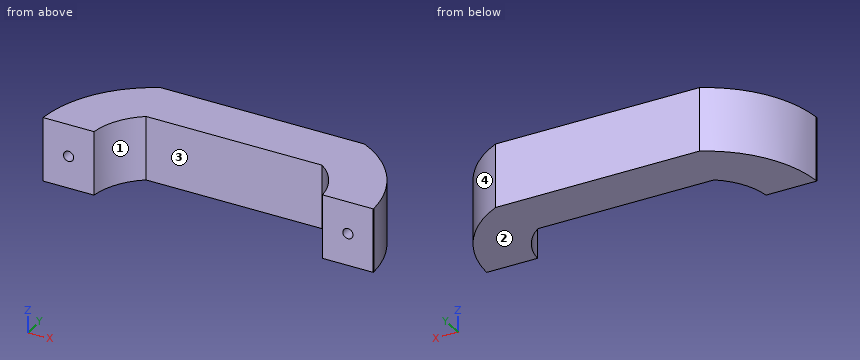
from build123d import *

# Parameters (mm, degrees)
BOSS_EXTRUDE1_DEPTH = 25
SKETCH3_R           = 2
CUT_EXTRUDE1_DEPTH  = 10


with BuildPart() as part:
    # Sketch2 → Boss-Extrude1 (new body)
    with BuildSketch(Plane.XY):
        with BuildLine():
            Line((-34.654096647, 18), (33.564112537, 18))
            Line((33.564112537, 18), (34.654096647, 18))
            ThreePointArc((34.654096647, 18), (41.754772696, 10.113790987), (44.967734696, 0))
            Line((44.967734696, 0), (64.929939713, 0))
            ThreePointArc((64.929939713, 0), (64.983093484, 0.336809111), (64.97700751, 0.677732359))
            ThreePointArc((64.97700751, 0.677732359), (57.505542276, 22.646902561), (40.105840234, 38))
            Line((40.105840234, 38), (33.564112537, 38))
            Line((33.564112537, 38), (-40.105840234, 38))
            ThreePointArc((-40.105840234, 38), (-57.505542276, 22.646902561), (-64.97700751, 0.677732359))
            ThreePointArc((-64.97700751, 0.677732359), (-65.02406211, 0.339344907), (-65.063625193, 0))
            Line((-65.063625193, 0), (-44.967734696, 0))
            ThreePointArc((-44.967734696, 0), (-41.754772696, 10.113790987), (-34.654096647, 18))
        make_face()
    extrude(amount=BOSS_EXTRUDE1_DEPTH)

    # Sketch3 → Cut-Extrude1 (cut)
    with BuildSketch(Plane.XZ):
        with Locations(Location((-55, 12.5, 0), (0, 0, 270))):
            Circle(SKETCH3_R)
        with Locations(Location((55, 12.5, 0), (0, 0, 90))):
            Circle(SKETCH3_R)
    extrude(amount=-CUT_EXTRUDE1_DEPTH, mode=Mode.SUBTRACT)


solid = part.part
Source: CAD feature listing. Evaluate the final solid. Frame: model axes, mm. Face numbers are marked on the shaded views. Give positions to 0.01 mm unless a question says otherwise; leave off trailing zeros. Order: outer loops, then holes, each group sorted by start corner. A loop starts at its lowest first (then second) coordinate and runs counter-clockwise, first axis right, second up. Notation, with made-up numbers: (41, -20.75) -> (81, -20.75) arc R19 ccw to (81, -7.75) -> close; hole circle Ø3 at (1.5, -15.5). An arc over 180 degrees is marked (long way). Write item = value, one per line.
Q1. Pin query (flat end, axial travel): pin 1 (8 mm diameter, centred on x = 27.5, y = 16.5, fed in from -Z); pin 2 (1.2 mm diameter, centred on x = 54, z = 13, fed in from -Y); pin 3 (8 mm diameter, centred on y = 5, z = 12.5, fed in from +X); pin 4 (12.5 mm diameter, centred on x = 8, z = 12.5, fed in from -Y). Return the tip coordinate at first contact, or that it passes through.
Data:
pin_1 = 0
pin_2 = 10
pin_3 = 64.95
pin_4 = 18
Q2. Cut plane B-B, the plane z = 12.5. Output: boundary loops of the cut face in (x, y).
Data:
outline = (-65.06, 0) -> (-57, 0) -> (-57, 10) -> (-53, 10) -> (-53, 0) -> (-44.97, 0) arc R25.13 cw to (-34.65, 18) -> (34.65, 18) arc R25.13 cw to (44.97, 0) -> (53, 0) -> (53, 10) -> (57, 10) -> (57, 0) -> (64.93, 0) arc R1.96 ccw to (64.98, 0.68) arc R45.13 ccw to (40.11, 38) -> (-40.11, 38) arc R45.13 ccw to (-64.98, 0.68) arc R15.45 ccw to start
Q3. Cut plane A-A, the plane y = 6.5. Output: boundary loops of the cut face in (x, z).
Data:
outline = (-64.2, 0) -> (-43.46, 0) -> (-43.46, 25) -> (-64.2, 25) -> close; (43.46, 0) -> (64.2, 0) -> (64.2, 25) -> (43.46, 25) -> close; hole circle Ø4 at (-55, 12.5); hole circle Ø4 at (55, 12.5)
Q4. Cut plane C-C, the plane x = 55. Output: boundary loops of the cut face in (y, z).
Data:
outline = (0, 0) -> (26.05, 0) -> (26.05, 25) -> (0, 25) -> (0, 14.5) -> (10, 14.5) -> (10, 10.5) -> (0, 10.5) -> close
Q5. Cut plane D-D, the plane y = 33. Output: boundary loops of the cut face in (x, z), and give its area (3 significant figures).
Data:
outline = (-47.97, 0) -> (47.97, 0) -> (47.97, 25) -> (-47.97, 25) -> close
area = 2,400 mm^2
Q6. Pull-direction query (X, two-part tool) for the marked faces 1, 2, 3 and 4; classes: released by +X, released by -X, zero draft, split by the parting line, or undercut.
Data:
face_1 = undercut
face_2 = zero draft
face_3 = undercut
face_4 = released by +X
Q7. Material intervals for line 1 (X direction, y = 2, z = 12.5); line 2 (Y direction, x = -2.5, z = 19.5); line 3 (Z direction, x = 55, y = 5.5), sorted ascending. Write a range as from..to.
Data:
line_1 = -64.87..-57, -53..-44.7, 44.7..53, 57..64.87
line_2 = 18..38
line_3 = 0..10.5, 14.5..25
